Design review of the part shown in the three views and the two pictorial views. Dimensions are in mm from the part's minimum x, y and z. A direction names the side the tool comes from. Coordinates: 2 decimals unless noted, no trailing zeros. Loops run counter-clockwise (first coordinate to the right, second up) from the corner with the lowest first, then second, coordinate; pieces in that order, holes last. Notation, with made-up numbers: (37.25, -14.75) -> (95.25, -14.75) arc R22 cw to (95.25, 4.25) -> close; hole circle Ø5 at (-33.5, -23). An arc over 180 degrees is marked (long way). Answer in a Markdown table with one row per item.
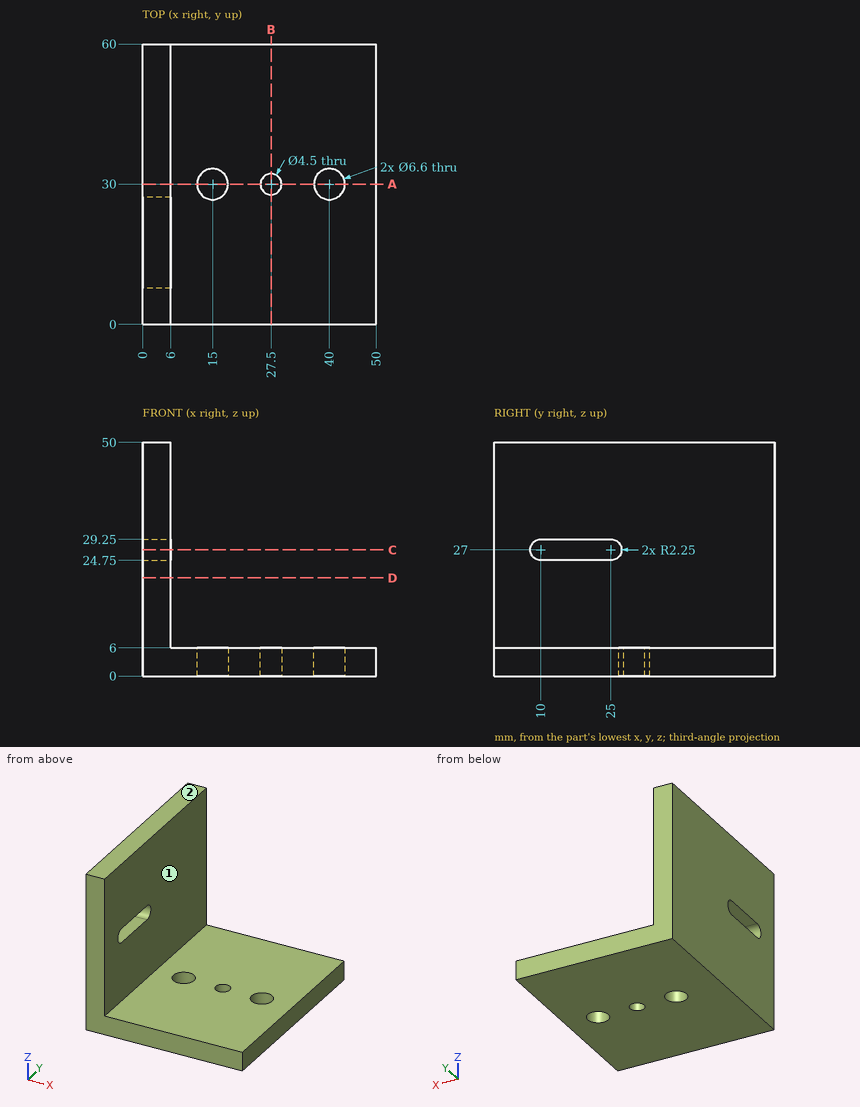
Item 1: For L1, parallel to Y at x = 27.5, z = 1.8; L2, parallel to Y at x = 15, z = 3.5; L3, parallel to X at y = 39.5, z = 40, list the stretches that pass through material, from the lowest coordinate up.
Worked answers:
| item | result |
|---|---|
| L1 | 0 to 27.75, 32.25 to 60 |
| L2 | 0 to 26.7, 33.3 to 60 |
| L3 | 0 to 6 |
Item 2: Take a section at D-D, the plane z = 21. State the section outline as (x, y) points, and give its area (3 significant figures).
Worked answers:
| item | result |
|---|---|
| outline | (0, 0) -> (6, 0) -> (6, 60) -> (0, 60) -> close |
| area | 360 mm² |
Item 3: For the marked faces 1 and 2, list the 3-axis set-ups (+Z, -Z, +X, -X, +Y, -Y) from which the entire face can be reached by the end or side of a thin tool; tool diameter is ignored.
Worked answers:
| item | result |
|---|---|
| face 1 | +Z, +X, +Y, -Y |
| face 2 | +Z, +X, -X, +Y, -Y |
Item 4: Take a section at C-C, the plane z = 27. State the section outline as (x, y) points, and give its area (3 significant figures).
Worked answers:
| item | result |
|---|---|
| outline | (0, 0) -> (6, 0) -> (6, 7.75) -> (0, 7.75) -> close; (0, 27.25) -> (6, 27.25) -> (6, 60) -> (0, 60) -> close |
| area | 243 mm² |
Item 5: Take a section at A-A, the plane y = 30. State the section outline as (x, z) points, and give its area (3 significant figures).
Worked answers:
| item | result |
|---|---|
| outline | (0, 0) -> (11.7, 0) -> (11.7, 6) -> (6, 6) -> (6, 50) -> (0, 50) -> close; (18.3, 0) -> (25.25, 0) -> (25.25, 6) -> (18.3, 6) -> close; (29.75, 0) -> (36.7, 0) -> (36.7, 6) -> (29.75, 6) -> close; (43.3, 0) -> (50, 0) -> (50, 6) -> (43.3, 6) -> close |
| area | 458 mm² |
Item 6: Insertion check: pin 1 (1.5 mm diameter, centred on y = 22.5, z = 26.5, fed in from -X); pin 2 (8 mm diameter, centred on x = 35, y = 14.5, fed in from +Z); pin 3 (1 mm diameter, centred on y = 12.5, z = 32.5, fed in from +X). Each pin has a flat end and moves straight along its axis. Give the tip position at first contact, or say it passes through.
Worked answers:
| item | result |
|---|---|
| pin 1 | through |
| pin 2 | z = 6 |
| pin 3 | x = 6 |
Item 7: Take a section at B-B, the plane x = 27.5. State the section outline as (y, z) points.
Worked answers:
| item | result |
|---|---|
| outline | (0, 0) -> (27.75, 0) -> (27.75, 6) -> (0, 6) -> close; (32.25, 0) -> (60, 0) -> (60, 6) -> (32.25, 6) -> close |
